from build123d import *

# Parameters (mm, degrees)
CUT_EXTRUDE1_DEPTH      = 55.559600438
CUT_EXTRUDE1_DEPTH_BACK = 55.559600438
SKETCH3_W               = 31.496031496
SKETCH3_H               = 31.496031496
CUT_EXTRUDE2_DEPTH      = 55.263283798
SKETCH6_R               = 7.6
CUT_EXTRUDE3_DEPTH      = 55.550435379


with BuildPart() as part:
    # Sketch1 → Revolve1 (revolve)
    with BuildSketch(Plane.XY):
        with BuildLine():
            Line((0, 31.5), (0, -31.5))
            ThreePointArc((0, -31.5), (-31.5, 0), (0, 31.5))
        make_face()
    revolve(axis=Axis((0, 31.5, 0), (0, -1, 0)))

    # Sketch2 → Cut-Extrude1 (cut, two sides: drawn at the far end of the back side and taken through both)
    with BuildSketch(Plane(origin=(0, 0, 0), x_dir=(1, 0, 0), z_dir=(0, 1, 0)).offset(-CUT_EXTRUDE1_DEPTH_BACK)):
        with BuildLine():
            Line((-0.5, 31.496031496), (-0.5, 0.5))
            Line((-0.5, 0.5), (-31.496031496, 0.5))
            ThreePointArc((-31.496031496, 0.5), (22.273863607, -22.273863607), (-0.5, 31.496031496))
        make_face()
    extrude(amount=CUT_EXTRUDE1_DEPTH + CUT_EXTRUDE1_DEPTH_BACK, mode=Mode.SUBTRACT)

    # Sketch3 → Cut-Extrude2 (cut, through all)
    with BuildSketch(Plane(origin=(-0.5, 0, 0), x_dir=(0, 0, -1), z_dir=(1, 0, 0))):
        with Locations((15.748015748, -15.748015748)):
            Rectangle(SKETCH3_W, SKETCH3_H)
    extrude(amount=-CUT_EXTRUDE2_DEPTH, mode=Mode.SUBTRACT)

    # Sketch6 → Cut-Extrude3 (cut, through all)
    with BuildSketch(Plane.XZ):
        Circle(SKETCH6_R)
    extrude(amount=-CUT_EXTRUDE3_DEPTH, mode=Mode.SUBTRACT)


solid = part.part
Here's how the part is built. I have some questions about the finished solid (model axes, mm). Coordinates: 2 decimals unless noted, no trailing zeros. Order: outer loops, then holes, each group sorted by start corner. A loop starts at its lowest first (then second) coordinate and runs counter-clockwise, first axis right, second up.
Item 1: I need wall thicknesses on line 1 (Z direction, x = -6, y = 20); line 2 (Y direction, x = -25, z = -9); line 3 (Y direction, x = -14, z = -2). Which ranges of each line are inside material? Lowest first, please.
Result sheet:
line 1: z = -23.58 to -4.66
line 2: y = 0 to 16.92
line 3: y = 0 to 28.15
Item 2: If we section it at D-D on y = 24: List the corners of the cut face in (x, z) for me, plus the area to 3 significant figures.
Result sheet:
outline: (-20.4, -0.5) arc R20.4 ccw to (-0.5, -20.4) - (-0.5, -7.58) arc R7.6 cw to (-7.58, -0.5) - close
area: 269 mm2
Item 3: If we section it at C-C on x = -3.5: List the corners of the cut face in (y, z) for me.
Result sheet:
outline: (0, -31.3) arc R31.3 ccw to (30.57, -6.75) - (0, -6.75) - close
Item 4: If we section it at A-A on y = 16.5: List the corners of the cut face in (x, z) for me.
Result sheet:
outline: (-26.83, -0.5) arc R26.83 ccw to (-0.5, -26.83) - (-0.5, -7.58) arc R7.6 cw to (-7.58, -0.5) - close
Item 5: If we section it at B-B on z = -5: List the corners of the cut face in (x, y) for me, plus the area to 3 significant figures.
Result sheet:
outline: (-31.1, 0) - (-5.72, 0) - (-5.72, 30.57) arc R31.1 ccw to start
area: 583 mm2
Item 6: For P1, Ø6, axis at y = 15.5, z = -9, coming from the -X side; P2, Ø5, axis at y = 20.5, z = -11, coming from the -X side; P3, Ø5, axis at x = -4, y = 13.5, coming from the -Z side, each with a flat end and sliding along its axis, tell me the tip position at first contact or that it passes through.
Result sheet:
P1: stops at x = -27.74
P2: stops at x = -23.69
P3: stops at z = -29.29
